```python
from build123d import *

# Parameters (mm, degrees)
BOSS_EXTRUDE1_DEPTH = 34.5
SKETCH3_R           = 15
CUT_EXTRUDE1_DEPTH  = 7
SKETCH4_W           = 7.5
SKETCH4_H           = 11
CUT_EXTRUDE2_DEPTH  = 58.5
SKETCH5_R           = 4.75
CUT_EXTRUDE3_DEPTH  = 14
SKETCH6_W           = 1
SKETCH6_H           = 11
CUT_EXTRUDE4_DEPTH  = 58.5
CUT_EXTRUDE5_REACH  = 53
SKETCH7_R           = 3
SKETCH8_R           = 1.75
CUT_EXTRUDE6_DEPTH  = 3


with BuildPart() as part:
    # Sketch1 → Boss-Extrude1 (new body)
    with BuildSketch(Plane.XY):
        Polygon((-9.056756757, 11), (31.443243243, 11), (31.443243243, 0), (39.943243243, 0), (39.943243243, 2), (33.443243243, 2), (33.443243243, 20), (-11.056756757, 20), (-11.056756757, 2), (-17.556756757, 2), (-17.556756757, 0), (-9.056756757, 0), align=None)
    extrude(amount=BOSS_EXTRUDE1_DEPTH)

    # Sketch3 → Cut-Extrude1 (cut)
    with BuildSketch(Plane(origin=(0, 20, 0), x_dir=(1, 0, 0), z_dir=(0, 1, 0))):
        with Locations((21.693243243, -17.25)):
            Circle(SKETCH3_R)
    extrude(amount=-CUT_EXTRUDE1_DEPTH, mode=Mode.SUBTRACT)

    # Sketch4 → Cut-Extrude2 (cut, through all)
    with BuildSketch(Plane.ZY.offset(17.556756757)):
        with Locations((3.75, 5.5)):
            Rectangle(SKETCH4_W, SKETCH4_H)
        with Locations((30.75, 5.5)):
            Rectangle(SKETCH4_W, SKETCH4_H)
    extrude(amount=-CUT_EXTRUDE2_DEPTH, mode=Mode.SUBTRACT)

    # Sketch5 → Cut-Extrude3 (cut, through all)
    with BuildSketch(Plane(origin=(0, 13, 0), x_dir=(1, 0, 0), z_dir=(0, 1, 0))):
        with Locations((21.693243243, -17.25)):
            Circle(SKETCH5_R)
    extrude(amount=-CUT_EXTRUDE3_DEPTH, mode=Mode.SUBTRACT)

    # Sketch6 → Cut-Extrude4 (cut, through all)
    with BuildSketch(Plane(origin=(39.943243243, 0, 0), x_dir=(0, 0, -1), z_dir=(1, 0, 0))):
        with Locations((-17.25, 5.5)):
            Rectangle(SKETCH6_W, SKETCH6_H)
    extrude(amount=-CUT_EXTRUDE4_DEPTH, mode=Mode.SUBTRACT)

    # Sketch7 → Cut-Extrude5 (cut, up to next)
    with BuildSketch(Plane.ZY.offset(11.056756757), mode=Mode.PRIVATE) as cut_extrude5_sk1:
        with Locations((17.75, 16.5)):
            Circle(SKETCH7_R)
    cut_extrude5_tool1 = extrude(cut_extrude5_sk1.sketch, amount=-CUT_EXTRUDE5_REACH, mode=Mode.PRIVATE) & part.part
    add(cut_extrude5_tool1.solids().sort_by_distance((-11.056757, 16.5, 17.75))[0], mode=Mode.SUBTRACT)

    # Sketch8 → Cut-Extrude6 (cut, through all)
    with BuildSketch(Plane(origin=(0, 2, 0), x_dir=(1, 0, 0), z_dir=(0, 1, 0))):
        with Locations((-13.306756757, -12.25)):
            Circle(SKETCH8_R)
        with Locations((-13.306756757, -22.25)):
            Circle(SKETCH8_R)
        with Locations((35.693243243, -22.25)):
            Circle(SKETCH8_R)
        with Locations((35.693243243, -12.25)):
            Circle(SKETCH8_R)
    extrude(amount=-CUT_EXTRUDE6_DEPTH, mode=Mode.SUBTRACT)


solid = part.part
```
Input: part model. Units: mm. Frame: model coordinates. A direction names the side the tool comes from. Round coordinates to 2 decimals unless told otherwise and drop trailing zeros. Write each loop counter-clockwise with the first axis right and the second up, starting at its lowest first coordinate (ties: lowest second). Pieces come first, ordered by that corner, then holes. Notation, with made-up numbers: (-18, 25) -> (37, 25) arc R13 cw to (37, 29) -> close; hole circle Ø10 at (4.5, 86.25). An arc over 180 degrees is marked (long way). Answer as CSV lines item,"result".
1. Contact query for flat-ended pins moving along their axis: P1, Ø3, axis at y = 14, z = 25, coming from the -X side; P2, Ø5, axis at x = -14, z = 21.5, coming from the +Y side; P3, Ø10, axis at x = -1.5, z = 25.5, coming from the -Y side. Output: stop coordinate, or through.
Geometry says:
P1,"stops at x = -11.06"
P2,"stops at y = 2"
P3,"stops at y = 11"
2. Ray query, L1, parallel to X at y = 11.7, z = 17.25; L2, parallel to X at y = 7, z = 26.5; L3, parallel to X at y = 1, z = 22. Return the intervals inside material, ascending. Write a range as [from, to].
Geometry says:
L1,"x = [-11.06, 16.94], [26.44, 33.44]"
L2,"x = [-11.06, -9.06], [31.44, 33.44]"
L3,"x = [-17.56, -15.04], [-11.57, -9.06], [31.44, 33.96], [37.43, 39.94]"
3. Mould query, pull axis Z, two halves, no side actions, for faces 5 (the flat face through (-15.3, 0, 12.1)), 6 (the flat face through (33, 3, 27)), 7 (the flat face through (33, 3, 16.75)). Classes: +Z half, -Z half, draft (parallel to the pull), parting line (faces both ways), or undercut.
Geometry says:
face 5,"draft"
face 6,"+Z half"
face 7,"undercut"
4. Section D-D (z = 28). Return the cut outline in (x, y), plus the area to 3 significant figures.
Geometry says:
outline,"(-11.06, 11) -> (33.44, 11) -> (33.44, 20) -> (32.15, 20) -> (32.15, 13) -> (11.23, 13) -> (11.23, 20) -> (-11.06, 20) -> close"
area,"254 mm^2"
5. Section C-C (x = 5). Return the cut outline in (y, z), plus the area to 3 significant figures.
Geometry says:
outline,"(11, 0) -> (20, 0) -> (20, 34.5) -> (11, 34.5) -> close; hole circle Ø6 at (16.5, 17.75)"
area,"282 mm^2"
6. Reachability of faces 1 (the flat face through (-11.057, 13, 17)), 2 (the flat face through (37.5, 2, 11)), 3 (the flat face through (-10.5, 3, 7.5)), 4 (the flat face through (31.443, 6, 22)) from +Z, -Z, +X, -X, +Y, -Y: full face, straight path, thin tool, end or side. Return the list, or none.
Geometry says:
face 1,"+Z, -Z, -X, +Y"
face 2,"+Z, -Z, +X, +Y"
face 3,"-Z, +X, -X, -Y"
face 4,"+Z, -Z, -Y"
7. Section A-A (y = 15.25). Return the cut outline in (x, z).
Geometry says:
outline,"(-11.06, 0) -> (33.44, 0) -> (33.44, 7.93) arc R15 cw to (6.86, 15.02) -> (-11.06, 15.02) -> close; (-11.06, 20.48) -> (7.04, 20.48) arc R15 cw to (33.44, 26.57) -> (33.44, 34.5) -> (-11.06, 34.5) -> close"
8. Section B-B (z = 19). Return the cut outline in (x, y), plus the area to 3 significant figures.
Geometry says:
outline,"(-17.56, 0) -> (-9.06, 0) -> (-9.06, 11) -> (17.28, 11) -> (17.28, 13) -> (6.8, 13) -> (6.8, 13.77) -> (-11.06, 13.77) -> (-11.06, 2) -> (-17.56, 2) -> close; (-11.06, 19.23) -> (6.8, 19.23) -> (6.8, 20) -> (-11.06, 20) -> close; (26.11, 11) -> (31.44, 11) -> (31.44, 0) -> (39.94, 0) -> (39.94, 2) -> (33.44, 2) -> (33.44, 13) -> (26.11, 13) -> close"
area,"169 mm^2"
